Print and shaded views of the part. All mm, measured from the part's lowest x, y and z. A direction names the side the tool comes from. Round coordinates to 2 decimals unless told otherwise and drop trailing zeros. Order: outer loops, then holes, each group sorted by start corner. A loop starts at its lowest first (then second) coordinate and runs counter-clockwise, first axis right, second up. Notation, with made-up numbers: (-10.75, 68) - (35.25, 68) arc R26 ccw to (35.25, 86) - close; hole circle Ø5 at (86.5, 48). An arc over 180 degrees is marked (long way). Write item = value, one per line.
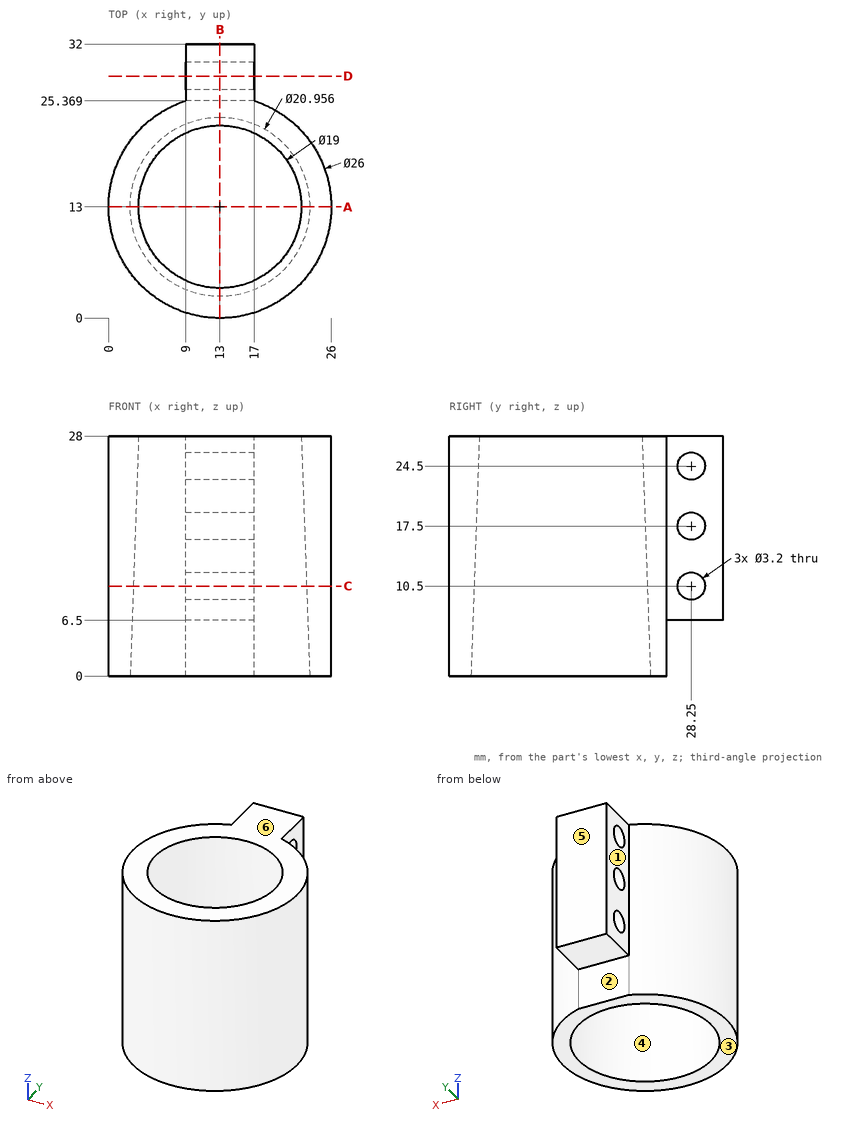
(1) Probe line 1 along Y through (x, z) = (14.25, 17.5); line 2 along Y through (x, z) = (12, 10.5); line 3 along Y through (x, z) = (15.75, 5.25) (1 decimal). List the from-to ranges inside material, lowest first.
Solved:
line_1 = 0.06 to 3.21, 22.79 to 26.65, 29.85 to 32
line_2 = 0.04 to 2.94, 23.06 to 26.65, 29.85 to 32
line_3 = 0.3 to 3.1, 22.9 to 25.4
(2) Band-saw the part on B-B on x = 13. List the corners of the cut face in (y, z).
Solved:
outline = (0, 0) - (2.52, 0) - (3.5, 28) - (0, 28) - close; (22.5, 28) - (23.48, 0) - (25.37, 0) - (25.37, 6.5) - (32, 6.5) - (32, 28) - close; hole circle Ø3.2 at (28.25, 10.5); hole circle Ø3.2 at (28.25, 17.5); hole circle Ø3.2 at (28.25, 24.5)
(3) Pull direction Y, two halves, no side cores. Call the marked faces 4, 5 and 6: released by +Y, released by -Y, zero draft, split by the parting line, or undercut.
Solved:
face_4 = undercut
face_5 = released by +Y
face_6 = zero draft
(4) Drop flat-ended pins along their axis: pin 1 (10 mm diameter, centred on y = 4, z = 7, fed in from +X); pin 2 (2.5 mm diameter, centred on y = 28.25, z = 10.5, fed in from +X); pin 3 (7.5 mm diameter, centred on x = 12, y = 29.5, fed in from -Z); pin 4 (8 mm diameter, centred on x = 8, z = 11.5, fed in from -Y). Give the stop position or say it passes through.
Solved:
pin_1 = 25.37
pin_2 = through
pin_3 = 6.5
pin_4 = 0.04
(5) Band-saw the part on D-D on y = 28.25. List the corners of the cut face in (x, z).
Solved:
outline = (9, 6.5) - (17, 6.5) - (17, 8.9) - (9, 8.9) - close; (9, 12.1) - (17, 12.1) - (17, 15.9) - (9, 15.9) - close; (9, 19.1) - (17, 19.1) - (17, 22.9) - (9, 22.9) - close; (9, 26.1) - (17, 26.1) - (17, 28) - (9, 28) - close
(6) Band-saw the part on C-C on z = 10.5. List the corners of the cut face in (x, y), plus the area to 3 significant figures.
Solved:
outline = (9, 25.37) arc R13 ccw (long way) to (17, 25.37) - (17, 26.65) - (9, 26.65) - close; (9, 29.85) - (17, 29.85) - (17, 32) - (9, 32) - close; hole circle Ø20.22 at (13, 13)
area = 234 mm²
(7) Tool access for the marked faces 1, 2 and 3: list every direction of +Z, -Z, +X, -X, +Y, -Y with a clear straight run to the whole face (end or side of a thin tool).
Solved:
face_1 = +Z, -Z, -X, +Y
face_2 = -Z, +X, -X, +Y
face_3 = -Z, +X, -X, +Y, -Y
(8) Band-saw the part on A-A on y = 13. List the corners of the cut face in (x, z), plus the area to 3 significant figures.
Solved:
outline = (0, 0) - (2.52, 0) - (3.5, 28) - (0, 28) - close; (22.5, 28) - (23.48, 0) - (26, 0) - (26, 28) - close
area = 169 mm²
